```python
from build123d import *

# Parameters (mm, degrees)
ESQUISSE1_W             = 2.5
ESQUISSE1_H             = 10
BOSS_EXTRU_1_DEPTH      = 7
BOSS_EXTRU_2_DEPTH      = 3
BOSS_EXTRU_2_DEPTH_BACK = 10
ENL_V_MAT_EXTRU_1_REACH = 44.024
ESQUISSE4_4_W           = 7
ESQUISSE4_4_H           = 9.399494937
ENL_V_MAT_EXTRU_4_DEPTH = 3
ENL_V_START             = -13
ESQUISSE4_W             = 7
ESQUISSE4_H             = 9.399494937
ENL_V_MAT_EXTRU_2_DEPTH = 3
CHANFREIN1_SIZE         = 3
CONG_1_R                = 1
ESQUISSE5_R             = 4.8
ENL_V_MAT_EXTRU_5_DEPTH = 1
ESQUISSE6_R             = 2.5
ESQUISSE6_R_2           = 2
ENL_V_MAT_EXTRU_6_DEPTH = 42.047043387
CHANFREIN2_SIZE         = 1


with BuildPart() as part:
    # Esquisse1 → Boss.-Extru.1 (new body)
    with BuildSketch(Plane.XY):
        Polygon((-8, 6), (-16, 6), (-16, 1), (-16, -9), (-16, -24), (-21, -24), (-7.5, -34), (0, -34), (0, 0), (-2, 0), align=None)
        Polygon((2, 0), (0, 0), (0, -34), (7.5, -34), (21, -24), (16, -24), (16, -9), (16, 1), (16, 6), (8, 6), align=None)
        with Locations((17.25, -4)):
            Rectangle(ESQUISSE1_W, ESQUISSE1_H)
        with Locations((-17.25, -4)):
            Rectangle(ESQUISSE1_W, ESQUISSE1_H)
    extrude(amount=BOSS_EXTRU_1_DEPTH)

    # Esquisse2 → Boss.-Extru.2 (add, two sides: drawn at the far end of the back side and taken through both)
    with BuildSketch(Plane.XY.offset(7).offset(-BOSS_EXTRU_2_DEPTH_BACK)):
        Polygon((16, -14), (-16, -14), (-16, -24), (-21, -24), (-7.5, -34), (7.5, -34), (21, -24), (16, -24), align=None)
    extrude(amount=BOSS_EXTRU_2_DEPTH + BOSS_EXTRU_2_DEPTH_BACK)

    # Esquisse3 → Enlèv. mat.-Extru.1 (cut, up to next)
    with BuildSketch(Plane(origin=(0, 0, -3), x_dir=(-1, 0, 0), z_dir=(0, 0, -1)), mode=Mode.PRIVATE) as enl_v_mat_extru_1_sk1:
        Polygon((-11, -0.899494937), (-3.5, -8.399494937), (-3.5, -23.399494937), (-11, -15.899494937), align=None)
    enl_v_mat_extru_1_tool1 = extrude(enl_v_mat_extru_1_sk1.sketch, amount=-ENL_V_MAT_EXTRU_1_REACH, mode=Mode.PRIVATE) & part.part
    # Esquisse3 → Enlèv. mat.-Extru.1 (cut, up to next)
    with BuildSketch(Plane(origin=(0, 0, -3), x_dir=(-1, 0, 0), z_dir=(0, 0, -1)), mode=Mode.PRIVATE) as enl_v_mat_extru_1_sk2:
        Polygon((11, -15.899494937), (11, -0.899494937), (3.5, -8.399494937), (3.5, -23.399494937), align=None)
    enl_v_mat_extru_1_tool2 = extrude(enl_v_mat_extru_1_sk2.sketch, amount=-ENL_V_MAT_EXTRU_1_REACH, mode=Mode.PRIVATE) & part.part
    add(enl_v_mat_extru_1_tool1.solids().sort_by_distance((7.25, -12.149495, -3))[0], mode=Mode.SUBTRACT)
    add(enl_v_mat_extru_1_tool2.solids().sort_by_distance((-7.25, -12.149495, -3))[0], mode=Mode.SUBTRACT)

    # Esquisse4<4> → Enlèv. mat.-Extru.4 (cut)
    with BuildSketch(Plane(origin=(0, 0, -3), x_dir=(-1, 0, 0), z_dir=(0, 0, -1))):
        with Locations((0, -18.699747469)):
            Rectangle(ESQUISSE4_4_W, ESQUISSE4_4_H)
    extrude(amount=-ENL_V_MAT_EXTRU_4_DEPTH, mode=Mode.SUBTRACT)

    # Esquisse4 → Enlèv. mat.-Extru.2 (cut)
    with BuildSketch(Plane(origin=(0, 0, -3), x_dir=(-1, 0, 0), z_dir=(0, 0, -1)).offset(ENL_V_START)):
        with Locations((0, -18.699747469)):
            Rectangle(ESQUISSE4_W, ESQUISSE4_H)
    extrude(amount=ENL_V_MAT_EXTRU_2_DEPTH, mode=Mode.SUBTRACT)

    # Chanfrein1
    chanfrein1_edges = [part.edges().sort_by_distance(p)[0] for p in [
        (-13.5, -14, 0),
        (-13.5, -14, 7),
        (13.5, -14, 0),
        (13.5, -14, 7),
    ]]
    chamfer(chanfrein1_edges, length=CHANFREIN1_SIZE - 0.0001)  # a hair under: the kernel refuses the full size

    # Congé1
    cong_1_edges = [part.edges().sort_by_distance(p)[0] for p in [
        (11, -15.899494937, 3.5),
        (11, -0.899494937, 3.5),
        (-11, -0.899494937, 3.5),
        (-11, -15.899494937, 3.5),
        (-21, -24, 3.5),
        (21, -24, 3.5),
    ]]
    fillet(cong_1_edges, radius=CONG_1_R)

    # Esquisse5 → Enlèv. mat.-Extru.5 (cut)
    with BuildSketch(Plane.XZ.offset(34)):
        with Locations(Location((0, 3.5, 0), (0, 0, 270))):
            Circle(ESQUISSE5_R)
    extrude(amount=-ENL_V_MAT_EXTRU_5_DEPTH, mode=Mode.SUBTRACT)

    # Esquisse6 → Enlèv. mat.-Extru.6 (cut, through all)
    with BuildSketch(Plane.XY.offset(10)):
        with Locations((-10, -24)):
            Circle(ESQUISSE6_R)
        with Locations((0, -28.5)):
            Circle(ESQUISSE6_R_2)
        with Locations(Location((10, -24, 0), (0, 0, 180))):
            Circle(ESQUISSE6_R)
    extrude(amount=-ENL_V_MAT_EXTRU_6_DEPTH, mode=Mode.SUBTRACT)

    # Chanfrein2
    chanfrein2_edges = [part.edges().sort_by_distance(p)[0] for p in [
        (0, -34, -3),
        (0, -34, 10),
    ]]
    chamfer(chanfrein2_edges, length=CHANFREIN2_SIZE)


solid = part.part
```
Design review of the part built by this model. Coordinates are the model's own, in mm. A direction names the side the tool comes from. Round coordinates to 2 decimals unless told otherwise and drop trailing zeros. Write each loop counter-clockwise with the first axis right and the second up, starting at its lowest first coordinate (ties: lowest second). Pieces come first, ordered by that corner, then holes.
Item 1: For faces 4 (the flat face through (-6.4, -5.5, 3.5)), 5 (the flat face through (-17, -24, 3)), 6 (the flat face through (0, -33, 4)), 7 (the flat face through (5, 3, 3)), list the 3-axis set-ups (+Z, -Z, +X, -X, +Y, -Y) from which the entire face can be reached by the end or side of a thin tool; tool diameter is ignored.
Item 2: We need section C-C on x = -10. Write out the cut boundary in (y, z), and give its area (3 significant figures).
Item 3: The part is to be moulded in two halves that separate along Y. For faces 1 (the cylindrical face through (-0.434, -30.452, 3.591)), 2 (the flat face through (12, 6, 3)), 3 (the flat face through (0, -25, -3)), say which applies: +Y half, -Y half, draft (parallel to the pull), parting line (faces both ways), or undercut.
Item 4: For probe 1 along X at (y, z) = (-9.5, 1); probe 2 along X at (y, z) = (-15, -2.25); probe 3 along Y at (x, z) = (8, 4), list the stretches that pass through material, from the lowest coordinate up.
Item 5: We need section D-D on y = -25. Write out the cut boundary in (x, z).
Item 6: We need section B-B on x = 0. Write out the cut boundary in (y, z), and give its area (3 significant figures).
Item 7: Clearance check with flat-ended pins moving along their axes: pin 1 Ø4 at (y, z) = (0, 4.5) entering from -X; pin 2 Ø12 at (x, y) = (-12.5, -5.5) entering from +Z; pin 3 Ø3.5 at (x, z) = (-0.5, -1) entering from +Y; pin 4 Ø4 at (x, y) = (-10, -24) entering from +Z. State where each tip first meets the part, or that it passes through.
Item 8: We need section A-A on y = 2. Write out the cut boundary in (x, z), and give its area (3 significant figures).
Returned:
1. face 4: +Z, -Z
1. face 5: +Z, -Z, -X
1. face 6: -Y
1. face 7: +Z, -Z, +Y
2. outline: (-32.15, -3) - (-26.5, -3) - (-26.5, 10) - (-32.15, 10) - close; (-21.5, -3) - (-16.9, -3) - (-16.9, 10) - (-21.5, 10) - close; (-2.31, 0) - (6, 0) - (6, 7) - (-2.31, 7) - close
2. area: 191 mm2
3. face 1: undercut
3. face 2: +Y half
3. face 3: draft
4. probe 1: x = -16 to -11, -3.5 to 3.5, 11 to 16
4. probe 2: x = -16 to -11, 11 to 16
4. probe 3: y = -33.63 to -25.5, -22.5 to -18.9, -3.9 to 6
5. outline: (-18.97, -3) - (-12.29, -3) - (-12.29, 10) - (-18.97, 10) - close; (-7.71, -3) - (7.71, -3) - (7.71, 10) - (-7.71, 10) - close; (12.29, -3) - (18.97, -3) - (18.97, 10) - (12.29, 10) - close
6. outline: (-34, -2) - (-33, -3) - (-30.5, -3) - (-30.5, 10) - (-33, 10) - (-34, 9) - (-34, 8.3) - (-33, 8.3) - (-33, -1.3) - (-34, -1.3) - close; (-26.5, -3) - (-23.4, -3) - (-23.4, 0) - (0, 0) - (0, 7) - (-23.4, 7) - (-23.4, 10) - (-26.5, 10) - close
6. area: 239 mm2
7. pin 1: stops at x = -18.5
7. pin 2: stops at z = 7.5
7. pin 3: stops at y = 0
7. pin 4: passes through
8. outline: (-16, 0) - (-4, 0) - (-4, 7) - (-16, 7) - close; (4, 0) - (16, 0) - (16, 7) - (4, 7) - close
8. area: 168 mm2
